```python
from build123d import *

# Parameters (mm, degrees)
SKETCH1_R           = 13
SKETCH1_R_2         = 1.05
SKETCH1_R_3         = 1.044026492
BOSS_EXTRUDE1_DEPTH = 1.6


with BuildPart() as part:
    # Sketch1 → Boss-Extrude1 (new body)
    with BuildSketch(Plane.XY):
        Polygon((72.39, -58.58), (72.4, -84.71), (81.44, -92.56), (81.43, -146.54), (213.35, -146.53), (213.35, -92.55), (222.39, -84.73), (222.39, -58.58), align=None)
        with Locations((149.01, -100.02)):
            Circle(SKETCH1_R, mode=Mode.SUBTRACT)
        with Locations((202.46, -120.78)):
            Circle(SKETCH1_R_2, mode=Mode.SUBTRACT)
        with Locations((202.48, -138.37)):
            Circle(SKETCH1_R_2, mode=Mode.SUBTRACT)
        with Locations((92.18, -138.41)):
            Circle(SKETCH1_R_3, mode=Mode.SUBTRACT)
        with Locations((92.17, -120.83)):
            Circle(SKETCH1_R_2, mode=Mode.SUBTRACT)
        with Locations((131.334, -117.57)):
            Circle(SKETCH1_R_2, mode=Mode.SUBTRACT)
        with Locations((166.686, -117.57)):
            Circle(SKETCH1_R_2, mode=Mode.SUBTRACT)
        with Locations((173.01, -93.57)):
            Circle(SKETCH1_R_2, mode=Mode.SUBTRACT)
        with Locations((125.01, -93.57)):
            Circle(SKETCH1_R_2, mode=Mode.SUBTRACT)
    extrude(amount=BOSS_EXTRUDE1_DEPTH)


solid = part.part
```
The model under review builds one solid part; all positions refer to its coordinate system, in mm. Round coordinates to 2 decimals unless told otherwise and drop trailing zeros. Order: outer loops, then holes, each group sorted by start corner. A loop starts at its lowest first (then second) coordinate and runs counter-clockwise, first axis right, second up. Notation, with made-up numbers: M -39.5,64 L -20.5,64 A25 cw -20.5,101 Z; hole C 33.5,60.5 d8. An arc over 180 degrees is marked long. Use a Markdown table: item, result.
1) Insertion check: pin 1 (1.3 mm diameter, centred on x = 92.17, y = -120.83, fed in from -Z). The pin has a flat end and moves straight along its axis. Give the tip position at first contact, or say it passes through.
Report:
| item | result |
|---|---|
| pin 1 | through |
2) Consider section B-B (z = 0.65). Give the number of separate pieces and of enclosed holes in the cut face, then the cut area to 3 significant figures.
Report:
| item | result |
|---|---|
| separate pieces | 1 |
| enclosed holes | 9 |
| area | 11,600 mm^2 |
3) Wall thickness on line 1 along X through (y, z) = (-138.41, 1); line 2 along Y through (x, z) = (202.46, 0.7); line 3 along Y through (x, z) = (92.17, 0.9): over which ranges is each line inside the solid? List them lowest first. Write a range as [from, to].
Report:
| item | result |
|---|---|
| line 1 | [81.43, 91.14], [93.22, 201.43], [203.53, 213.35] |
| line 2 | [-146.53, -139.42], [-137.32, -121.83], [-119.73, -58.58] |
| line 3 | [-146.54, -139.45], [-137.37, -121.88], [-119.78, -58.58] |
4) Consider section A-A (y = -106). Write out the cut boundary in (x, z).
Report:
| item | result |
|---|---|
| outline | M 81.44,0 L 137.47,0 L 137.47,1.6 L 81.44,1.6 Z; M 160.55,0 L 213.35,0 L 213.35,1.6 L 160.55,1.6 Z |
5) Consider section C-C (y = -88.5). Write out the cut boundary in (x, z), then the cut area to 3 significant figures.
Report:
| item | result |
|---|---|
| outline | M 76.76,0 L 142.99,0 L 142.99,1.6 L 76.76,1.6 Z; M 155.03,0 L 218.03,0 L 218.03,1.6 L 155.03,1.6 Z |
| area | 207 mm^2 |
6) Draft analysis for pull direction X (two halves, no side actions). For faces 1 (the face through (161.02, -105, 0.79)), 2 (the face through (217.8, -88.7, 0.8)), 3 (the face through (163, -102, 1.6)), state which applies: released by +X, released by -X, zero draft, split by the parting line, or undercut.
Report:
| item | result |
|---|---|
| face 1 | undercut |
| face 2 | released by +X |
| face 3 | zero draft |
